Read the model definition and answer for the solid it produces. Units are mm, in the model's axes. A direction names the side the tool comes from. Give positions to 0.01 mm unless a question says otherwise; leave off trailing zeros. Write each loop counter-clockwise with the first axis right and the second up, starting at its lowest first coordinate (ties: lowest second). Pieces come first, ordered by that corner, then holes. Notation, with made-up numbers: (84.25, 76) -> (89.25, 76) arc R24 ccw to (89.25, 115) -> close; hole circle Ø4 at (3, 6.25). An arc over 180 degrees is marked (long way). Use a Markdown table: item, result.
from build123d import *

# Parameters (mm, degrees)
BOSS_EXTRUDE1_DEPTH = 5
SKETCH2_R           = 1.25
SKETCH2_W           = 12
SKETCH2_H           = 23
CUT_EXTRUDE1_DEPTH  = 5


with BuildPart() as part:
    # Sketch1 → Boss-Extrude1 (new body)
    with BuildSketch(Plane(origin=(0, 0, 0), x_dir=(1, 0, 0), z_dir=(0, 1, 0))):
        Polygon((-10, 20), (-10, -20), (-3.5, -20), (-3.5, -15), (3.5, -15), (3.5, -20), (10, -20), (10, 20), (3.5, 20), (3.5, 25), (-3.5, 25), (-3.5, 20), align=None)
    extrude(amount=BOSS_EXTRUDE1_DEPTH)

    # Sketch2 → Cut-Extrude1 (cut)
    with BuildSketch(Plane(origin=(0, 5, 0), x_dir=(1, 0, 0), z_dir=(0, 1, 0))):
        with Locations(Location((0, 17, 0), (0, 0, 270))):
            Circle(SKETCH2_R)
        with Locations(Location((0, -12, 0), (0, 0, 270))):
            Circle(SKETCH2_R)
        with Locations((0, 2.5)):
            Rectangle(SKETCH2_W, SKETCH2_H)
    extrude(amount=-CUT_EXTRUDE1_DEPTH, mode=Mode.SUBTRACT)


solid = part.part
Item 1: A cutting plane is placed at B-B (z = 8). Give the vertices of the cut face in (x, y).
Return value:
| item | result |
|---|---|
| outline | (-10, 0) -> (-6, 0) -> (-6, 5) -> (-10, 5) -> close; (6, 0) -> (10, 0) -> (10, 5) -> (6, 5) -> close |
Item 2: A cutting plane is placed at A-A (x = 5.5). Give the vertices of the cut face in (y, z).
Return value:
| item | result |
|---|---|
| outline | (0, -20) -> (5, -20) -> (5, -14) -> (0, -14) -> close; (0, 9) -> (5, 9) -> (5, 20) -> (0, 20) -> close |
Item 3: A cutting plane is placed at C-C (y = 0.8). Give the vertices of the cut face in (x, z), then the cut area to 3 significant figures.
Return value:
| item | result |
|---|---|
| outline | (-10, -20) -> (-3.5, -20) -> (-3.5, -25) -> (3.5, -25) -> (3.5, -20) -> (10, -20) -> (10, 20) -> (3.5, 20) -> (3.5, 15) -> (-3.5, 15) -> (-3.5, 20) -> (-10, 20) -> close; hole (-6, -14) -> (6, -14) -> (6, 9) -> (-6, 9) -> close; hole circle Ø2.5 at (0, -17); hole circle Ø2.5 at (0, 12) |
| area | 514 mm^2 |
Item 4: Straight lines are drawn through the part: line 1 along X through (y, z) = (1.9, -17); line 2 along X through (y, z) = (3.8, 3); line 3 along Z through (x, y) = (5, 2.3). For each, find the intervals that lie inside material, in ascending order. Write a range as [from, to].
Return value:
| item | result |
|---|---|
| line 1 | [-10, -1.25], [1.25, 10] |
| line 2 | [-10, -6], [6, 10] |
| line 3 | [-20, -14], [9, 20] |
Item 5: For a pull along Z with two mould halves and no side action, classify faces 1 (the face through (0.05, 2.54, 10.75)), 2 (the face through (-7, 2, 20)), 3 (the face through (3.5, 2, 17)) as +Z half, -Z half, draft (parallel to the pull), parting line (faces both ways), or undercut.
Return value:
| item | result |
|---|---|
| face 1 | undercut |
| face 2 | +Z half |
| face 3 | draft |
Item 6: A tool of negligible diameter and unlimited length cuts with its end or side. For faces 4 (the face through (3.5, 2, -22)), 5 (the face through (0, 3, 9)), 6 (the face through (-3.5, 2, 18)), from which of +Z, -Z, +X, -X, +Y, -Y can it reach the whole face along a straight path? Write none if from no direction.
Return value:
| item | result |
|---|---|
| face 4 | -Z, +X, +Y, -Y |
| face 5 | +Y, -Y |
| face 6 | +Z, +Y, -Y |
Item 7: Each of these flat-tipped pins is pushed along its axis until it touches: P1, Ø2.5, axis at y = 3.5, z = -23, coming from the +X side; P2, Ø3, axis at x = 0.5, y = 3, coming from the +Z side; P3, Ø2.5, axis at y = 3, z = -22, coming from the -X side. Where does it stop, or does it pass through?
Return value:
| item | result |
|---|---|
| P1 | x = 3.5 |
| P2 | z = 15 |
| P3 | x = -3.5 |
Item 8: A cutting plane is placed at D-D (x = 0). Give the vertices of the cut face in (y, z).
Return value:
| item | result |
|---|---|
| outline | (0, -25) -> (5, -25) -> (5, -18.25) -> (0, -18.25) -> close; (0, -15.75) -> (5, -15.75) -> (5, -14) -> (0, -14) -> close; (0, 9) -> (5, 9) -> (5, 10.75) -> (0, 10.75) -> close; (0, 13.25) -> (5, 13.25) -> (5, 15) -> (0, 15) -> close |
